Verification items for the finished model (mm, model axes). Give positions to 0.01 mm unless a question says otherwise; leave off trailing zeros. Loops run counter-clockwise (first coordinate to the right, second up) from the corner with the lowest first, then second, coordinate; pieces in that order, holes last. Notation, with made-up numbers: M 45,-36 L 52,-36 A33 ccw 52,-7 Z; hole C 28,8.25 d6. An arc over 180 degrees is marked long. Use a Markdown table: item, result.
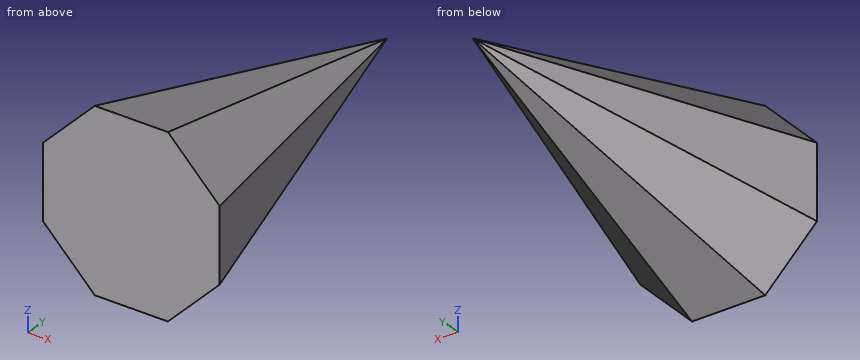
from build123d import *


with BuildPart() as part:
    # Sketch1 → Loft1 section 0
    with BuildSketch(Plane(origin=(0, 0, 0), x_dir=(1, 0, 0), z_dir=(0, 1, 0)), mode=Mode.PRIVATE) as loft1_s0:
        Polygon((2.071067812, -5), (5, -2.071067812), (5, 2.071067812), (2.071067812, 5), (-2.071067812, 5), (-5, 2.071067812), (-5, -2.071067812), (-2.071067812, -5), align=None)
    loft([Vertex(0, 20, 0), loft1_s0.sketch])


solid = part.part
(1) Cross-section at B-B on x = 1.5. Record the cut outline in (y, z).
Results below:
| item | result |
|---|---|
| outline | M 0,-5 L 5.51,-3.62 L 14,-0.62 L 14,0.62 L 5.51,3.62 L 0,5 Z |
(2) Cross-section at D-D on y = 10. Record the cut outline in (x, z).
Results below:
| item | result |
|---|---|
| outline | M -2.5,-1.04 L -1.04,-2.5 L 1.04,-2.5 L 2.5,-1.04 L 2.5,1.04 L 1.04,2.5 L -1.04,2.5 L -2.5,1.04 Z |
(3) Gauge pin test, flat ends, axial feed: P1, Ø1.5, axis at y = 2.5, z = 3.5, coming from the -X side; P2, Ø5, axis at y = 8, z = -2.5, coming from the -X side; P3, Ø4, axis at x = -3.5, y = 2, coming from the +Z side. Record the tip position at first contact, or that the pin passes through.
Results below:
| item | result |
|---|---|
| P1 | x = -3.48 |
| P2 | x = -3.57 |
| P3 | z = 4.83 |
(4) Cross-section at A-A on y = 12.75. Record the cut outline in (x, z), then the cut area to 3 significant figures.
Results below:
| item | result |
|---|---|
| outline | M -1.81,-0.75 L -0.75,-1.81 L 0.75,-1.81 L 1.81,-0.75 L 1.81,0.75 L 0.75,1.81 L -0.75,1.81 L -1.81,0.75 Z |
| area | 10.9 mm^2 |
(5) Cross-section at C-C on z = 0.75. Record the cut outline in (x, y), then the cut area to 3 significant figures.
Results below:
| item | result |
|---|---|
| outline | M -5,0 L 5,0 L 1.81,12.76 L 0.31,17 L -0.31,17 L -1.81,12.76 Z |
| area | 95.9 mm^2 |
(6) Material ranges on line 1 (X direction, y = 5.75, z = 0.5); line 2 (Z direction, x = 0.5, y = 16.75); line 3 (Z direction, x = 0, y = 4.25), recorded low to high.
Results below:
| item | result |
|---|---|
| line 1 | -3.56 to 3.56 |
| line 2 | -0.65 to 0.65 |
| line 3 | -3.94 to 3.94 |
